Model file for the job. Use its own axes, mm. Face numbers are marked on the shaded views. A direction names the side the tool comes from. Give positions to 0.01 mm unless a question says otherwise; leave off trailing zeros. Loops run counter-clockwise (first coordinate to the right, second up) from the corner with the lowest first, then second, coordinate; pieces in that order, holes last. Notation, with made-up numbers: (55, 10.5) - (71, 10.5) arc R24 ccw to (71, 26.5) - close; hole circle Ø10 at (36.5, 15.25). An arc over 180 degrees is marked (long way). Use a Markdown table: item, result.
from build123d import *

# Parameters (mm, degrees)
SKETCH_5_R          = 2
SKETCH_5_R_2        = 2.55
EXTRUDE_3_DEPTH     = 15
FILLET_4_R          = 4
SKETCH_6_R          = 6.4
EXTRUDE_4_DEPTH     = 22.45
SKETCH_7_R          = 6.5
CUT_EXTRUDE_1_DEPTH = 4.7
CUT_EXTRUDE_START   = -4.7
SKETCH_8_R          = 6.5
CUT_EXTRUDE_2_DEPTH = 4.7
SKETCH_9_W          = 7.5
SKETCH_9_H          = 50
CUT_EXTRUDE_3_DEPTH = 60.938467095
SKETCH_10_R         = 3.55
CUT_EXTRUDE_4_DEPTH = 1.5


with BuildPart() as part:
    # 草图5 → 凸台-拉伸3 (new body)
    with BuildSketch(Plane.XY):
        with BuildLine():
            Line((15.516814201, 7.002212297), (7.384422843, 8.091371903))
            ThreePointArc((7.384422843, 8.091371903), (5.833974337, 8.425935573), (4.355928265, 9.00143816))
            ThreePointArc((4.355928265, 9.00143816), (-6.069854623, 7.947129347), (-9.830420232, -1.833804259))
            ThreePointArc((-9.830420232, -1.833804259), (-9.664128327, -3.411197812), (-9.749336047, -4.995042206))
            Line((-9.749336047, -4.995042206), (-11.383433357, -17.196301568))
            ThreePointArc((-11.383433357, -17.196301568), (-11.717997026, -18.746750074), (-12.293499614, -20.224796146))
            ThreePointArc((-12.293499614, -20.224796146), (-4.619495141, -34.492228828), (6.538358778, -22.746920152))
            ThreePointArc((6.538358778, -22.746920152), (6.372066873, -21.169526599), (6.457274593, -19.585682205))
            Line((6.457274593, -19.585682205), (7.194690182, -14.07964606))
            ThreePointArc((7.194690182, -14.07964606), (8.731350099, -11.431767797), (11.690265423, -10.646017769))
            Line((11.690265423, -10.646017769), (13.127433564, -10.838495653))
            Line((13.127433564, -10.838495653), (15.516814201, 7.002212297))
        make_face()
        Circle(SKETCH_5_R, mode=Mode.SUBTRACT)
        with Locations((-3.292061454, -24.580724411)):
            Circle(SKETCH_5_R_2, mode=Mode.SUBTRACT)
    extrude(amount=EXTRUDE_3_DEPTH)

    # 圆角4
    # the kernel refuses this fillet: 4 mm, written as the material it takes off along each edge
    with BuildSketch(Plane(origin=(-19.660840464, -3.667608519, 15), x_dir=(0.9830420232040514, 0.18338042593168238, 0), z_dir=(-0.18338042593168238, 0.9830420232040514, 0))) as fillet_4_piece_1:
        with BuildLine():
            CenterArc((10 + FILLET_4_R, FILLET_4_R), FILLET_4_R, 180, 90)
            Line((10 + FILLET_4_R, 0), (10, 0))
            Line((10, 0), (10, FILLET_4_R))
        make_face()
    revolve(axis=Axis((-19.660840464, -3.667608519, 15), (0, 0, -1)), revolution_arc=18.194872339, mode=Mode.SUBTRACT)
    with BuildSketch(Plane(origin=(25.428318618, 5.67477861, 0), x_dir=(0, 0, 1), z_dir=(-0.9911504416884656, 0.132743368726124, 0))) as fillet_4_piece_2:
        with BuildLine():
            CenterArc((FILLET_4_R, -FILLET_4_R), FILLET_4_R, 90, 90)
            Line((0, -FILLET_4_R), (0, 0))
            Line((0, 0), (FILLET_4_R, 0))
        make_face()
    extrude(amount=18.205002002, mode=Mode.SUBTRACT)
    with BuildSketch(Plane(origin=(11.690265423, -10.646017769, 0), x_dir=(0, 0, 1), z_dir=(0.9911504416883519, -0.13274336872697298, 0))) as fillet_4_piece_3:
        with BuildLine():
            CenterArc((FILLET_4_R, -FILLET_4_R), FILLET_4_R, 90, 90)
            Line((0, -FILLET_4_R), (0, 0))
            Line((0, 0), (FILLET_4_R, 0))
        make_face()
    extrude(amount=11.45, mode=Mode.SUBTRACT)
    with BuildSketch(Plane(origin=(11.159291948, -14.610619535, 0), x_dir=(-0.9911504416882816, 0.13274336872749704, 0), z_dir=(-0.13274336872749704, -0.9911504416882816, 0))) as fillet_4_piece_4:
        with BuildLine():
            CenterArc((4 + FILLET_4_R, -FILLET_4_R), FILLET_4_R, 90, 90)
            Line((4 + FILLET_4_R, 0), (4, 0))
            Line((4, 0), (4, -FILLET_4_R))
        make_face()
    revolve(axis=Axis((11.159291948, -14.610619535, 0), (0, 0, -1)), revolution_arc=90, mode=Mode.SUBTRACT)
    with BuildSketch(Plane(origin=(6.457274593, -19.585682205, 0), x_dir=(0, 0, 1), z_dir=(0.13274336872730183, 0.9911504416883078, 0))) as fillet_4_piece_5:
        with BuildLine():
            CenterArc((FILLET_4_R, -FILLET_4_R), FILLET_4_R, 90, 90)
            Line((0, -FILLET_4_R), (0, 0))
            Line((0, 0), (FILLET_4_R, 0))
        make_face()
    extrude(amount=5.555197186, mode=Mode.SUBTRACT)
    with BuildSketch(Plane(origin=(16.368779012, -20.913115892, 0), x_dir=(-0.3768153606688204, -0.9262883913576953, 0), z_dir=(0.9262883913576953, -0.3768153606688204, 0))) as fillet_4_piece_6:
        with BuildLine():
            CenterArc((10.000000001 + FILLET_4_R, -FILLET_4_R), FILLET_4_R, 90, 90)
            Line((10.000000001 + FILLET_4_R, 0), (10.000000001, 0))
            Line((10.000000001, 0), (10.000000001, -FILLET_4_R))
        make_face()
    revolve(axis=Axis((16.368779012, -20.913115892, 0), (0, 0, -1)), revolution_arc=75.491592277, mode=Mode.SUBTRACT)
    with BuildSketch(Plane(origin=(-9.749336047, -4.995042206, 15), x_dir=(0, 0, -1), z_dir=(-0.13274336872713738, -0.9911504416883298, 0))) as fillet_4_piece_7:
        with BuildLine():
            CenterArc((FILLET_4_R, FILLET_4_R), FILLET_4_R, 180, 90)
            Line((0, FILLET_4_R), (0, 0))
            Line((0, 0), (FILLET_4_R, 0))
        make_face()
    extrude(amount=12.310199188, mode=Mode.SUBTRACT)
    with BuildSketch(Plane(origin=(-21.294937774, -15.868867881, 0), x_dir=(0.9911504416879034, -0.132743368730321, 0), z_dir=(0.132743368730321, 0.9911504416879034, 0))) as fillet_4_piece_8:
        with BuildLine():
            CenterArc((10 + FILLET_4_R, -FILLET_4_R), FILLET_4_R, 90, 90)
            Line((10 + FILLET_4_R, 0), (10, 0))
            Line((10, 0), (10, -FILLET_4_R))
        make_face()
    revolve(axis=Axis((-21.294937774, -15.868867881, 0), (0, 0, -1)), revolution_arc=75.491592288, mode=Mode.SUBTRACT)
    with BuildSketch(Plane(origin=(-9.749336047, -4.995042206, 0), x_dir=(0, 0, 1), z_dir=(-0.13274336872713738, -0.9911504416883298, 0))) as fillet_4_piece_9:
        with BuildLine():
            CenterArc((FILLET_4_R, -FILLET_4_R), FILLET_4_R, 90, 90)
            Line((0, -FILLET_4_R), (0, 0))
            Line((0, 0), (FILLET_4_R, 0))
        make_face()
    extrude(amount=12.310199188, mode=Mode.SUBTRACT)
    with BuildSketch(Plane(origin=(-19.660840464, -3.667608519, 0), x_dir=(0.9830420232040514, 0.18338042593168238, 0), z_dir=(-0.18338042593168238, 0.9830420232040514, 0))) as fillet_4_piece_10:
        with BuildLine():
            CenterArc((10 + FILLET_4_R, -FILLET_4_R), FILLET_4_R, 90, 90)
            Line((10 + FILLET_4_R, 0), (10, 0))
            Line((10, 0), (10, -FILLET_4_R))
        make_face()
    revolve(axis=Axis((-19.660840464, -3.667608519, 0), (0, 0, -1)), revolution_arc=18.194872339, mode=Mode.SUBTRACT)
    with BuildSketch(Plane(origin=(0, 0, 0), x_dir=(0.43559282651439474, 0.900143816003421, 0), z_dir=(0.900143816003421, -0.43559282651439474, 0))) as fillet_4_piece_11:
        with BuildLine():
            CenterArc((10 - FILLET_4_R, FILLET_4_R), FILLET_4_R, 270, 90)
            Line((10 - FILLET_4_R, 0), (10, 0))
            Line((10, 0), (10, FILLET_4_R))
        make_face()
    revolve(axis=Axis((0, 0, 0), (0, 0, 1)), revolution_arc=126.389744678, mode=Mode.SUBTRACT)
    with BuildSketch(Plane(origin=(8.71185653, 18.00287632, 0), x_dir=(-0.13274336873032264, -0.9911504416879031, 0), z_dir=(0.9911504416879031, -0.13274336873032264, 0))) as fillet_4_piece_12:
        with BuildLine():
            CenterArc((10 + FILLET_4_R, -FILLET_4_R), FILLET_4_R, 90, 90)
            Line((10 + FILLET_4_R, 0), (10, 0))
            Line((10, 0), (10, -FILLET_4_R))
        make_face()
    revolve(axis=Axis((8.71185653, 18.00287632, 0), (0, 0, -1)), revolution_arc=18.194872339, mode=Mode.SUBTRACT)
    with BuildSketch(Plane(origin=(-21.294937774, -15.868867881, 15), x_dir=(0.9911504416879034, -0.132743368730321, 0), z_dir=(0.132743368730321, 0.9911504416879034, 0))) as fillet_4_piece_13:
        with BuildLine():
            CenterArc((10 + FILLET_4_R, FILLET_4_R), FILLET_4_R, 180, 90)
            Line((10 + FILLET_4_R, 0), (10, 0))
            Line((10, 0), (10, FILLET_4_R))
        make_face()
    revolve(axis=Axis((-21.294937774, -15.868867881, 15), (0, 0, -1)), revolution_arc=75.491592288, mode=Mode.SUBTRACT)
    with BuildSketch(Plane(origin=(16.368779012, -20.913115892, 15), x_dir=(-0.3768153606688204, -0.9262883913576953, 0), z_dir=(0.9262883913576953, -0.3768153606688204, 0))) as fillet_4_piece_14:
        with BuildLine():
            CenterArc((10.000000001 + FILLET_4_R, FILLET_4_R), FILLET_4_R, 180, 90)
            Line((10.000000001 + FILLET_4_R, 0), (10.000000001, 0))
            Line((10.000000001, 0), (10.000000001, FILLET_4_R))
        make_face()
    revolve(axis=Axis((16.368779012, -20.913115892, 15), (0, 0, -1)), revolution_arc=75.491592277, mode=Mode.SUBTRACT)
    with BuildSketch(Plane(origin=(6.457274593, -19.585682205, 15), x_dir=(0, 0, -1), z_dir=(0.13274336872730183, 0.9911504416883078, 0))) as fillet_4_piece_15:
        with BuildLine():
            CenterArc((FILLET_4_R, FILLET_4_R), FILLET_4_R, 180, 90)
            Line((0, FILLET_4_R), (0, 0))
            Line((0, 0), (FILLET_4_R, 0))
        make_face()
    extrude(amount=5.555197186, mode=Mode.SUBTRACT)
    with BuildSketch(Plane(origin=(11.159291948, -14.610619535, 15), x_dir=(-0.9911504416882816, 0.13274336872749704, 0), z_dir=(-0.13274336872749704, -0.9911504416882816, 0))) as fillet_4_piece_16:
        with BuildLine():
            CenterArc((4 + FILLET_4_R, FILLET_4_R), FILLET_4_R, 180, 90)
            Line((4 + FILLET_4_R, 0), (4, 0))
            Line((4, 0), (4, FILLET_4_R))
        make_face()
    revolve(axis=Axis((11.159291948, -14.610619535, 15), (0, 0, -1)), revolution_arc=90, mode=Mode.SUBTRACT)
    with BuildSketch(Plane(origin=(11.690265423, -10.646017769, 15), x_dir=(0, 0, -1), z_dir=(0.9911504416883519, -0.13274336872697298, 0))) as fillet_4_piece_17:
        with BuildLine():
            CenterArc((FILLET_4_R, FILLET_4_R), FILLET_4_R, 180, 90)
            Line((0, FILLET_4_R), (0, 0))
            Line((0, 0), (FILLET_4_R, 0))
        make_face()
    extrude(amount=11.45, mode=Mode.SUBTRACT)
    with BuildSketch(Plane(origin=(25.428318618, 5.67477861, 15), x_dir=(0, 0, -1), z_dir=(-0.9911504416884656, 0.132743368726124, 0))) as fillet_4_piece_18:
        with BuildLine():
            CenterArc((FILLET_4_R, FILLET_4_R), FILLET_4_R, 180, 90)
            Line((0, FILLET_4_R), (0, 0))
            Line((0, 0), (FILLET_4_R, 0))
        make_face()
    extrude(amount=18.205002002, mode=Mode.SUBTRACT)
    with BuildSketch(Plane(origin=(8.71185653, 18.00287632, 15), x_dir=(-0.13274336873032264, -0.9911504416879031, 0), z_dir=(0.9911504416879031, -0.13274336873032264, 0))) as fillet_4_piece_19:
        with BuildLine():
            CenterArc((10 + FILLET_4_R, FILLET_4_R), FILLET_4_R, 180, 90)
            Line((10 + FILLET_4_R, 0), (10, 0))
            Line((10, 0), (10, FILLET_4_R))
        make_face()
    revolve(axis=Axis((8.71185653, 18.00287632, 15), (0, 0, -1)), revolution_arc=18.194872339, mode=Mode.SUBTRACT)
    with BuildSketch(Plane(origin=(0, 0, 15), x_dir=(0.43559282651439474, 0.900143816003421, 0), z_dir=(0.900143816003421, -0.43559282651439474, 0))) as fillet_4_piece_20:
        with BuildLine():
            CenterArc((10 - FILLET_4_R, -FILLET_4_R), FILLET_4_R, 0, 90)
            Line((10 - FILLET_4_R, 0), (10, 0))
            Line((10, 0), (10, -FILLET_4_R))
        make_face()
    revolve(axis=Axis((0, 0, 15), (0, 0, 1)), revolution_arc=126.389744678, mode=Mode.SUBTRACT)

    # 草图6 → 凸台-拉伸4 (add)
    with BuildSketch(Plane(origin=(14.322123882, -1.918141678, 0), x_dir=(0, 0, -1), z_dir=(0.9911504416882867, -0.13274336872745984, 0))):
        with Locations(Location((-7.5, 0, 0), (0, 0, 270))):
            Circle(SKETCH_6_R)
    extrude(amount=EXTRUDE_4_DEPTH)

    # 草图7 → 切除-拉伸1 (cut)
    with BuildSketch(Plane.XY.offset(15)):
        with Locations((-3.292061454, -24.580724411)):
            Circle(SKETCH_7_R)
    extrude(amount=-CUT_EXTRUDE_1_DEPTH, mode=Mode.SUBTRACT)

    # 草图8 → 切除-拉伸2 (cut)
    with BuildSketch(Plane(origin=(0, 0, 0), x_dir=(-1, 0, 0), z_dir=(0, 0, -1)).offset(CUT_EXTRUDE_START)):
        with Locations(Location((3.292061454, -24.580724411, 0), (0, 0, 180))):
            Circle(SKETCH_8_R)
    extrude(amount=CUT_EXTRUDE_2_DEPTH, mode=Mode.SUBTRACT)

    # 草图9 → 切除-拉伸3 (cut, through all)
    with BuildSketch(Plane(origin=(36.573451298, -4.898230306, 0), x_dir=(0, 0, -1), z_dir=(0.9911504416882867, -0.13274336872745987, 0))):
        with Locations((-3.75, -9.800195184)):
            Rectangle(SKETCH_9_W, SKETCH_9_H)
    extrude(amount=-CUT_EXTRUDE_3_DEPTH, mode=Mode.SUBTRACT)

    # 草图10 → 切除-拉伸4 (cut)
    with BuildSketch(Plane.XY.offset(15)):
        Circle(SKETCH_10_R)
    extrude(amount=-CUT_EXTRUDE_4_DEPTH, mode=Mode.SUBTRACT)


solid = part.part
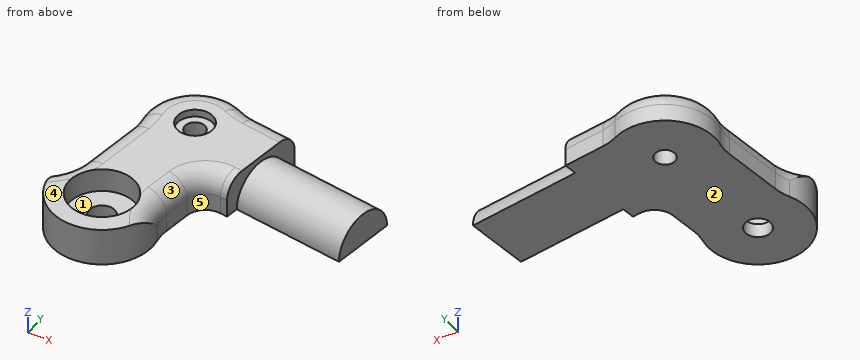
(1) 3-axis set-ups, long thin cutter, end or side, ignore diameter. For the marked faces 1 and 2: which of +Z, -Z, +X, -X, +Y, -Y reach the whole face in a straight line?
Computed:
| item | result |
|---|---|
| face 1 | +Z |
| face 2 | -Z, +X, -X, +Y, -Y |
(2) Drill centre lines: probe 1 along Y at (x, z) = (0, 10.9); probe 2 along Z at (x, y) = (-5.5, -28); probe 3 along X at (y, z) = (-1, 11.25). Where is each one in solid material? Low to high. Write a range as [from, to].
Computed:
| item | result |
|---|---|
| probe 1 | [-34.02, -30.19], [-18.98, -2], [2, 10] |
| probe 2 | [7.5, 10.3] |
| probe 3 | [-9.94, -1.73], [1.73, 37.1] |
(3) Slice it at A-A, the plane z = 9.25. Write the cut outline in (x, y), plus the area to 3 significant figures.
Computed:
| item | result |
|---|---|
| outline | (-12.29, -20.22) arc R10 ccw (long way) to (6.54, -22.75) arc R10 cw to (6.46, -19.59) - (7.19, -14.08) arc R4 cw to (11.69, -10.65) - (13.13, -10.84) - (13.5, -8.02) - (35.76, -11) - (37.39, 1.2) - (15.14, 4.18) - (15.52, 7) - (7.38, 8.09) arc R10 cw to (4.36, 9) arc R10 ccw to (-9.83, -1.83) arc R10 cw to (-9.75, -5) - (-11.38, -17.2) arc R10 cw to start; hole circle Ø5.1 at (-3.29, -24.58); hole circle Ø4 at (0, 0) |
| area | 1,120 mm² |
(4) Slice it at C-C, the plane y = -32. Write the cut outline in (x, z).
Computed:
| item | result |
|---|---|
| outline | (-10, 7.5) - (3.41, 7.5) - (3.41, 15) - (-10, 15) - close |
(5) Mould opens along X. For the marked faces 3, 4 and 5 say: pulls with the +X half, pulls with the -X half, needs draft (parallel to the pull), parting line crosses it, or undercut.
Computed:
| item | result |
|---|---|
| face 3 | pulls with the +X half |
| face 4 | needs draft |
| face 5 | undercut |
(6) Pin check, flat tips, straight feed: P1, Ø4, axis at x = -3.29, y = -24.58, coming from the -Z side; P2, Ø2, axis at y = -6, z = 9.5, coming from the +X side; P3, Ø1, axis at y = -11.5, z = 12, coming from the +X side; P4, Ø8, axis at x = -3.29, y = -24.58, coming from the +Z side. Stop position of each tip, or through.
Computed:
| item | result |
|---|---|
| P1 | through |
| P2 | x = 36.56 |
| P3 | x = 9.19 |
| P4 | z = 10.3 |
(7) Slice it at B-B, the plane x = 0. Write the cut outline in (y, z), plus the area to 3 significant figures.
Computed:
| item | result |
|---|---|
| outline | (-34.02, 7.5) - (-2, 7.5) - (-2, 13.5) - (-3.55, 13.5) - (-3.55, 15) - (-18.98, 15) - (-18.98, 10.3) - (-30.19, 10.3) - (-30.19, 15) - (-34.02, 15) - close; (2, 7.5) - (10, 7.5) - (10, 11) arc R4 ccw to (6, 15) - (3.55, 15) - (3.55, 13.5) - (2, 13.5) - close |
| area | 239 mm² |
